from build123d import *

# Parameters (mm, degrees)
F0_W     = 127
F0_H     = 76.2
F2_DEPTH = 76.2
F3_W     = 77.3548015118
F3_H     = 26.4147613198
F4_DEPTH = 88.138
F5_W     = 76.9804359138
F5_H     = 7.3428414762
F6_DEPTH = 93.98
F7_R     = 25.2764175419
F8_DEPTH = 142.494


with BuildPart() as f2:
    # F0 (on Front) → F2 (new body)
    with BuildSketch(Plane.XZ):
        with Locations((5.8183724284, 27.8661628202)):
            Rectangle(F0_W, F0_H)
    extrude(amount=F2_DEPTH)

    # F3 (on Front) → F4 (cut)
    with BuildSketch(Plane.XZ):
        with Locations((6.3353191733, 3.1585739926)):
            Rectangle(F3_W, F3_H)
    extrude(amount=F4_DEPTH, mode=Mode.SUBTRACT)

    # F5 (on face) → F6 (cut)
    with BuildSketch(Plane.XZ.offset(76.2)):
        with Locations((6.1481363744, -13.7202274054)):
            Rectangle(F5_W, F5_H)
    extrude(amount=-F6_DEPTH, mode=Mode.SUBTRACT)

    # F7 (on face) → F8 (cut)
    with BuildSketch(Plane.YZ.offset(69.3183724284)):
        with Locations((-38.1, 65.9661628202)):
            Circle(F7_R)
    extrude(amount=-F8_DEPTH, mode=Mode.SUBTRACT)


solid = f2.part
Geometry: final body of the model. Coordinates: model frame, mm. A direction names the side the tool comes from. Give positions to 0.01 mm unless a question says otherwise; leave off trailing zeros. Write each loop counter-clockwise with the first axis right and the second up, starting at its lowest first coordinate (ties: lowest second). Pieces come first, ordered by that corner, then holes. Notation, with made-up numbers: M -12.75,79.25 L 29.25,79.25 A13 ccw 29.25,86.25 Z; hole C -24.5,-32.75 d4. An arc over 180 degrees is marked long. Answer in a Markdown table with one row per item. Add a question column.
(1) Reachability of faces 4 (the flat face through (5, -6, 65.966)), 5 (the flat face through (-32.342, -39, 3)) from +Z, -Z, +X, -X, +Y, -Y: full face, straight path, thin tool, end or side. Return the list, or none.
(2) Section D-D on x = 61. Return loops of the section in (y, z), and give its area (3 significant figures).
(3) Section B-B on x = 27. Return loops of the section in (y, z).
(4) Mould query, pull axis Z, two halves, no side actions, for faces 1 (the flat face through (45.013, -38, 3)), 2 (the flat face through (69.318, -38, 19)), 3 (the flat face through (-45, -38, -10.234)). Classes: +Z half, -Z half, draft (parallel to the pull), parting line (faces both ways), or undercut.
(5) Section A-A on y = -38.1. Return loops of the section in (x, z).
(6) Ray query, line 1 (X direction, y = -70, z = -2); line 2 (Y direction, x = 28.5, z = 50.5); line 3 (Y direction, x = -6, z = 46). Return the intervals inside material, ascending.
(7) First-contact query: pin 1 (4 mm diameter, centred on x = 12.5, y = -45.5, fed in from +Z); pin 2 (23 mm diameter, centred on x = -3.5, y = -39.5, fed in from -Z). Flat tips, straight axial feed; report the tip coordinate or a pass-through.
(8) Section C-C on y = -60. Return loops of the section in (x, z), and give its area (3 significant figures).
Result set:
| question | item | result |
|---|---|---|
| 1 | face 4 | +Z, +X, -X, +Y, -Y |
| 1 | face 5 | -Z, +Y, -Y |
| 2 | outline | M -76.2,-10.23 L 0,-10.23 L 0,65.97 L -12.82,65.97 A25.28 cw -63.38,65.97 L -76.2,65.97 Z |
| 2 | area | 4,800 mm^2 |
| 3 | outline | M -76.2,16.37 L 0,16.37 L 0,65.97 L -12.82,65.97 A25.28 cw -63.38,65.97 L -76.2,65.97 Z |
| 4 | face 1 | undercut |
| 4 | face 2 | draft |
| 4 | face 3 | -Z half |
| 5 | outline | M -57.68,-10.23 L -32.34,-10.23 L -32.34,16.37 L 45.01,16.37 L 45.01,-10.05 L 44.64,-10.05 L 44.64,-10.23 L 69.32,-10.23 L 69.32,40.69 L -57.68,40.69 Z |
| 6 | line 1 | x = -57.68 to -32.34, 45.01 to 69.32 |
| 6 | line 2 | y = -76.2 to -58.09, -18.11 to 0 |
| 6 | line 3 | y = -76.2 to -53.6, -22.6 to 0 |
| 7 | pin 1 | stops at z = 42.5 |
| 7 | pin 2 | stops at z = 16.37 |
| 8 | outline | M -57.68,-10.23 L -32.34,-10.23 L -32.34,16.37 L 45.01,16.37 L 45.01,-10.05 L 44.64,-10.05 L 44.64,-10.23 L 69.32,-10.23 L 69.32,53.35 L -57.68,53.35 Z |
| 8 | area | 6,020 mm^2 |
